The listing builds one solid part. Answer for the finished solid, in the listing's coordinates (mm). Face numbers are marked on the shaded views. A direction names the side the tool comes from. Round coordinates to 2 decimals unless told otherwise and drop trailing zeros. Order: outer loops, then holes, each group sorted by start corner. A loop starts at its lowest first (then second) coordinate and runs counter-clockwise, first axis right, second up. Notation, with made-up numbers: (40.5, -9) - (71.5, -9) arc R32 ccw to (71.5, 19) - close; hole circle Ø9 at (86.5, 50.5). An arc over 180 degrees is marked (long way). One line per item, written item: value. Start each with the question number.
1. Section A-A, the plane y = 0 is taken. Give the vertices of the cut face in (x, z), then the cut area to 3 significant figures.
2. Flat-ended cylindrical pins translate along their axes: P1, Ø2.5, axis at x = -4.5, z = 2.5, coming from the +Y side; P2, Ø2, axis at x = -4, z = -3.5, coming from the +Y side; P3, Ø2, axis at x = 0.5, y = -9, coming from the -Z side. Find the tip coordinate at first contact, or state that the pin passes through.
3. Section D-D, the plane z = -3.5 is taken. Give the vertices of the cut face in (x, y), then the cut area to 3 significant figures.
4. A tool of negligible diameter and unlimited length cuts with its end or side. For the marked faces 1, 2, 3, 4 and 5, from which of +Z, -Z, +X, -X, +Y, -Y can it reach the whole face along a straight path? Write none if from no direction.
5. Section C-C, the plane z = 0 is taken. Give the vertices of the cut face in (x, y), then the cut area to 3 significant figures.
6. Straight lines are drawn through the part: line 1 (Z direction, x = 0.65, y = 0); line 2 (Y direction, x = 0.85, z = 4); line 3 (Z direction, x = 1, y = 7). For each, find the intervals that lie inside material, in ascending order.
7. For a pull along Z with two mould halves and no side action, classify the marked faces 6, 7, 8 and 9 as released by +Z, released by -Z, zero draft, split by the parting line, or undercut.
8. Section B-B, the plane x = -4.5 is taken. Give the vertices of the cut face in (y, z), then the cut area to 3 significant figures.
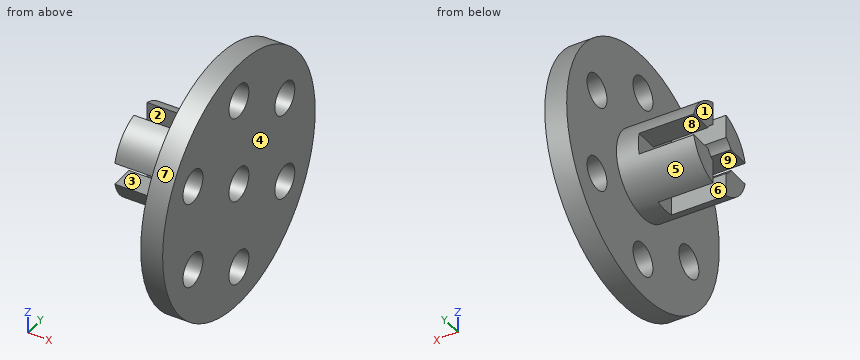
Autodesk Inventor part; units mm, degrees
ref_plane "YZ Plane" through (0, 0, 0) normal (1, 0, 0) x (0, 1, 0)
ref_plane "XZ Plane" through (0, 0, 0) normal (0, 1, 0) x (-1, 0, 0)
ref_plane "XY Plane" through (0, 0, 0) normal (0, 0, 1) x (1, 0, 0)
sketch "スケッチ1" plane through (0, 0, 0) normal (1, 0, 0) x (0, 1, 0)
  circle A0 centre (0, 0) radius 11.5
  dimension "d0" = 23
extrude "押し出し1" add sketch "スケッチ1" along normal blind 2
sketch "スケッチ4" plane through (0, 0, 0) normal (-1, 0, 0) x (0, 0, 1)
  circle A0 centre (0, 0) radius 4
  dimension "d22" = 8
extrude "押し出し2" add sketch "スケッチ4" along normal blind 7
sketch "スケッチ5" plane through (-7, 0, 0) normal (-1, 0, 0) x (0, 0, 1)
  line L0 (-4, 1) -> (4, 1)
  line L1 (4, 1) -> (4, -1)
  line L2 (4, -1) -> (-4, -1)
  line L3 (-4, -1) -> (-4, 1)
  line L4 (-1, 4) -> (1, 4)
  line L5 (1, 4) -> (1, -4)
  line L6 (1, -4) -> (-1, -4)
  line L7 (-1, -4) -> (-1, 4)
  circle A0 centre (0, 0) radius 4
  circle A1 centre (0, 0) radius 2
  point P0 (0, 4)
  point P1 (4, 0)
  point P2 (1, 0)
  point P3 (0, 1)
  point P4 (1, 1)
  point P5 (-1, 1)
  point P6 (-1, -1)
  point P7 (1, -1)
  point P8 (-1, 1.7321)
  point P9 (-1.7321, 1)
  point P10 (1.7321, 1)
  point P11 (1, 1.7321)
  point P12 (-1.7321, -1)
  point P13 (-1, -1.7321)
  point P14 (1, -1.7321)
  point P15 (1.7321, -1)
  dimension "d25" = 2
  dimension "d26" = 2
  dimension "d29" = 4
extrude "押し出し3" cut sketch "スケッチ5" against normal blind 5 contours L0 A0 L3 | L0 A1 L2 A0 | A0 L2 L3 | A1 L7 L0 | L0 L7 L2 A1 | A0 L5 A1 L7 | L7 L4 A0 | L7 A1 L5 L0 | L0 L5 L2 L7 | L2 L7 A1 | L4 L5 A0 | A0 L6 L7 | L7 A1 L5 A0 | L5 A1 L0 | L0 A1 L2 L5 | L2 L5 A1 L7 | A0 L5 L6 | L0 A0 L2 A1 | L2 A1 L5 | L0 L1 A0 | L1 L2 A0
sketch "スケッチ2" plane through (2, 0, 0) normal (1, 0, 0) x (0, 0, -1)
  point P0 (0, 0)
  point P1 (0, 0)
hole "穴1" at (2, 0, 0) direction (-1, 0, 0) diameter 3 end through all
sketch "スケッチ3" plane through (2, 0, 0) normal (1, 0, 0) x (0, 0, -1)
  point P0 (0, 0)
  point P1 (8, 0)
  point P2 (4, 6.9282)
  point P3 (-4, 6.9282)
  point P4 (-8, 0)
  point P5 (-4, -6.9282)
  point P6 (4, -6.9282)
  dimension "d12" = 360
  dimension "d14" = 16
hole "穴2" at (2, 0, -8) at (2, 6.9282, -4) at (2, 6.9282, 4) at (2, 0, 8) at (2, -6.9282, 4) at (2, -6.9282, -4) direction (-1, 0, 0) diameter 3 end through all
equation "\"d25\" = d26"
properties part number "CircleArm"
Answer list:
1. outline: (-2, -4) - (0, -4) - (0, -6.5) - (2, -6.5) - (2, -1.5) - (-2, -1.5) - close; (-2, 1.5) - (2, 1.5) - (2, 6.5) - (0, 6.5) - (0, 4) - (-2, 4) - close; (0, -11.5) - (2, -11.5) - (2, -9.5) - (0, -9.5) - close; (0, 9.5) - (2, 9.5) - (2, 11.5) - (0, 11.5) - close
1. area: 38.0 mm²
2. P1: stops at y = 3.8
2. P2: stops at y = 3.12
2. P3: stops at z = -8.26
3. outline: (-7, -1.94) - (0, -1.94) - (0, -5.51) - (2, -5.51) - (2, 5.51) - (0, 5.51) - (0, 1.94) - (-7, 1.94) - (-7, 1) - (-2, 1) - (-2, -1) - (-7, -1) - close; (0, -10.95) - (2, -10.95) - (2, -8.34) - (0, -8.34) - close; (0, 8.34) - (2, 8.34) - (2, 10.95) - (0, 10.95) - close
3. area: 49.6 mm²
4. face 1: +Z, -Z, -X, +Y, -Y
4. face 2: +Z, -Z, -X
4. face 3: -X, +Y, -Y
4. face 4: +Z, -Z, +X, +Y, -Y
4. face 5: -X
5. outline: (-2, -4) - (0, -4) - (0, -11.5) - (2, -11.5) - (2, -1.5) - (-2, -1.5) - close; (-2, 1.5) - (2, 1.5) - (2, 11.5) - (0, 11.5) - (0, 4) - (-2, 4) - close
5. area: 50.0 mm²
6. line 1: z = -11.5 to -9.5, -6.5 to -1.5, 1.5 to 6.5, 9.5 to 11.5
6. line 2: y = -10.78 to -8.43, -5.43 to 5.43, 8.43 to 10.78
6. line 3: z = -9.12 to -5.5, -2.5 to 2.5, 5.5 to 9.12
7. face 6: zero draft
7. face 7: split by the parting line
7. face 8: undercut
7. face 9: undercut
8. outline: (-3.87, -1) arc R4 ccw to (-1, -3.87) - (-1, -1.73) arc R2 cw to (-1.73, -1) - close; (-3.87, 1) - (-1.73, 1) arc R2 cw to (-1, 1.73) - (-1, 3.87) arc R4 ccw to start; (1, -3.87) arc R4 ccw to (3.87, -1) - (1.73, -1) arc R2 cw to (1, -1.73) - close; (1, 1.73) arc R2 cw to (1.73, 1) - (3.87, 1) arc R4 ccw to (1, 3.87) - close
8. area: 21.3 mm²
